```python
from build123d import *

# Parameters (mm, degrees)
F2_R = 1


# Not quite as in the source:
# - a fillet or chamfer that OpenCascade refuses, or shapes differently, is made with other operations: its cross-section is extruded or revolved along the edge and cut away or added


with BuildPart() as f1:
    # F0 (on Front) → F1 (revolve)
    with BuildSketch(Plane.XZ):
        Polygon((0, 50), (0, 0), (15, 0), (20.62, 28.1), (20.82, 29.1), (25, 50), align=None)
        Polygon((20.82, 29.1), (20.62, 28.1), (20.87, 28.1), (20.87, 29.1), align=None)
    revolve(axis=Axis((0, 0, 25), (0, 0, -1)))

    # F2
    f2_edges = [f1.edges().sort_by_distance(p)[0] for p in [
        (-15, 0, 0),
    ]]
    fillet(f2_edges, radius=F2_R)

    # F3: fillet of radius 0.5 on 2 edges, made by hand

    # F3_s1 → F3_t2 (revolve, cut)
    with BuildSketch(Plane.XZ):
        with BuildLine():
            ThreePointArc((20.62, 28.1), (20.8030127019, 28.2830127019), (20.87, 28.5330127019))
            Line((20.87, 28.5330127019), (20.88, 28.5330127019))
            Line((20.88, 28.5330127019), (20.88, 28.1))
            Line((20.88, 28.1), (20.87, 28.09))
            ThreePointArc((20.87, 28.09), (20.745, 28.09), (20.625, 28.091339746))
            Line((20.625, 28.091339746), (20.62, 28.1))
        make_face()
    revolve(axis=Axis((0, 0, 28.1), (0, 0, -1)), mode=Mode.SUBTRACT)

    # F3_s3 → F3_t4 (revolve, cut)
    with BuildSketch(Plane.XZ):
        with BuildLine():
            ThreePointArc((20.87, 28.8820550528), (20.8573397172, 28.9938584517), (20.82, 29.1))
            Line((20.82, 29.1), (20.829, 29.1043588989))
            ThreePointArc((20.829, 29.1043588989), (20.845, 29.11), (20.87, 29.11))
            Line((20.87, 29.11), (20.88, 29.1))
            Line((20.88, 29.1), (20.88, 28.8820550528))
            Line((20.88, 28.8820550528), (20.87, 28.8820550528))
        make_face()
    revolve(axis=Axis((0, 0, 29.1), (0, 0, -1)), mode=Mode.SUBTRACT)


solid = f1.part
```
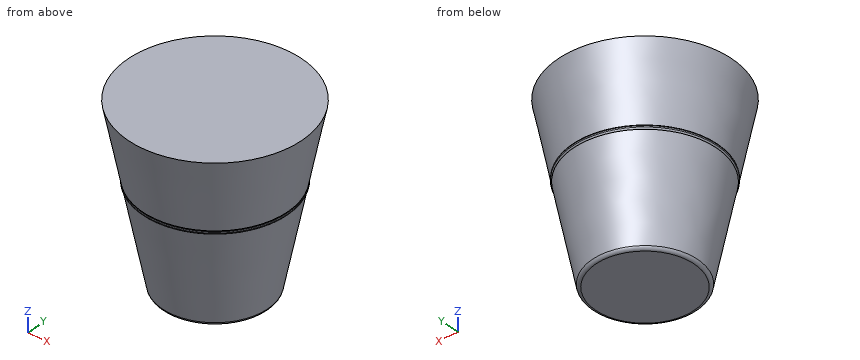
Geometry check sheet. Reference: the model listing, model coordinates, mm. Round coordinates to 2 decimals unless told otherwise and drop trailing zeros. Order: outer loops, then holes, each group sorted by start corner. A loop starts at its lowest first (then second) coordinate and runs counter-clockwise, first axis right, second up. Notation, with made-up numbers: (57.25, 26.25) -> (68.25, 26.25) arc R13 ccw to (68.25, 41.25) -> close; hole circle Ø1 at (4.25, -34.5). An arc over 180 degrees is marked (long way). Return JSON: item names as keys, results as strings. Group by question number.
Q1. Section check A-A, the plane y = 0. Record the boundary of the cut face in (x, z), plus the area to 3 significant figures.
Q2. Gauge pin test, flat ends, axial feed: pin 1 (2 mm diameter, centred on y = 9.5, z = 7.5, fed in from +X); pin 2 (1.5 mm diameter, centred on x = 5.5, z = 36, fed in from -Y); pin 3 (5 mm diameter, centred on x = -12.5, z = 21.5, fed in from -Y). Record the tip position at first contact, or that the pin passes through.
Q3. Section check D-D, the plane z = 33. Record the boundary of the cut face in (x, y).
Q4. Material ranges on probe 1 along Y at (x, z) = (-0.5, 15); probe 2 along Y at (x, z) = (7, 15); probe 3 along X at (y, z) = (0, 15), recorded low to high. Write a range as from..to.
Q5. Section check C-C, the plane z = 41. Record the boundary of the cut face in (x, y).
Numbers:
{
 "1": {"outline": "(-25, 50) -> (-20.82, 29.1) arc R0.5 ccw to (-20.87, 28.88) -> (-20.87, 28.53) arc R0.5 ccw to (-20.62, 28.1) -> (-15.16, 0.8) arc R1 ccw to (-14.18, 0) -> (14.18, 0) arc R1 ccw to (15.16, 0.8) -> (20.62, 28.1) arc R0.5 ccw to (20.87, 28.53) -> (20.87, 28.88) arc R0.5 ccw to (20.82, 29.1) -> (25, 50) -> close", "area": "2,000 mm^2"},
 "2": {"pin 1": "x = 14.19", "pin 2": "y = -21.75", "pin 3": "y = -16.62"},
 "3": {"outline": "circle Ø43.2 at (0, 0)"},
 "4": {"probe 1": "-17.99..17.99", "probe 2": "-16.58..16.58", "probe 3": "-18..18"},
 "5": {"outline": "circle Ø46.4 at (0, 0)"}
}
